```python
from build123d import *

# Parameters (mm, degrees)
SKETCH_R        = 4.075
PAD_DEPTH       = 10
SKETCH001_R     = 1.6
POCKET_DEPTH    = 10.501
POCKET001_DEPTH = 3
FILLET_R        = 3
FILLET001_R     = 1.5


with BuildPart() as part:
    # Sketch → Pad (new body)
    with BuildSketch(Plane.XY):
        with BuildLine():
            Line((20, -4.075), (20, -14.575))
            Line((20, -14.575), (-20, -14.575))
            Line((-20, -14.575), (-20, -4.075))
            Line((-20, -4.075), (-11.149975, -4.075))
            ThreePointArc((-11.149975, -4.075), (-8.268533, -2.881467), (-7.075, -2.5e-05))
            Line((-7.075, 0), (-7.075, -2.5e-05))
            ThreePointArc((7.075, 0), (0, 7.075), (-7.075, 0))
            Line((7.075, -2.5e-05), (7.075, 0))
            ThreePointArc((7.075, -2.5e-05), (8.268533, -2.881467), (11.149975, -4.075))
            Line((20, -4.075), (11.149975, -4.075))
        make_face()
        Circle(SKETCH_R, mode=Mode.SUBTRACT)
    extrude(amount=PAD_DEPTH)

    # Sketch001 (on Face6 of Pad) → Pocket (cut, through all)
    with BuildSketch(Plane(origin=(0, -4.075, 0), x_dir=(-1, 0, 0), z_dir=(0, 1, 0))):
        with Locations((-15.574988, 5)):
            Circle(SKETCH001_R)
        with Locations((15.574988, 5)):
            Circle(SKETCH001_R)
    extrude(amount=-POCKET_DEPTH, mode=Mode.SUBTRACT)

    # Sketch002 (on Face11 of Pocket) → Pocket001 (cut)
    with BuildSketch(Plane(origin=(0, -4.075, 0), x_dir=(-1, 0, 0), z_dir=(0, 1, 0))):
        Polygon((-15.574988, 8.233162), (-18.374988, 6.616581), (-18.374988, 3.383419), (-15.574988, 1.766838), (-12.774988, 3.383419), (-12.774988, 6.616581), align=None)
        Polygon((15.574988, 8.233162), (12.774988, 6.616581), (12.774988, 3.383419), (15.574988, 1.766838), (18.374988, 3.383419), (18.374988, 6.616581), align=None)
    extrude(amount=-POCKET001_DEPTH, mode=Mode.SUBTRACT)

    # Fillet
    fillet_edges = [part.edges().sort_by_distance(p)[0] for p in [
        (-20, -9.325, 0),
        (-20, -9.325, 10),
        (20, -9.325, 0),
        (20, -9.325, 10),
    ]]
    fillet(fillet_edges, radius=FILLET_R)

    # Fillet001
    fillet001_edges = [part.edges().sort_by_distance(p)[0] for p in [
        (-4.075, 0, 10),
        (-4.075, 0, 0),
    ]]
    fillet(fillet001_edges, radius=FILLET001_R)


solid = part.part
```
Read the model definition and answer for the solid it produces. Units are mm, in the model's axes. A direction names the side the tool comes from. Give positions to 0.01 mm unless a question says otherwise; leave off trailing zeros. Write each loop counter-clockwise with the first axis right and the second up, starting at its lowest first coordinate (ties: lowest second). Pieces come first, ordered by that corner, then holes. Notation, with made-up numbers: M 87.25,66.5 L 92.25,66.5 A9 ccw 92.25,76.5 Z; hole C 28.25,71 d7. An arc over 180 degrees is marked long. Put each result on its own line as item: value. Start each with the question number.
1. Each of these flat-tipped pins is pushed along its axis until it touches: pin 1 Ø1 at (y, z) = (-10, 9) entering from -X; pin 2 Ø4.5 at (x, z) = (-15, 4) entering from +Y (3 decimals); pin 3 Ø4.5 at (x, z) = (16, 5) entering from +Y (3 decimals). Where does it stop, or does it pass through?
2. For a pull along Z with two mould halves and no side action, classify faces 6 (the flat face through (0, -8, 10)), 7 (the flat face through (-20, -9, 5)), 8 (the flat face through (-14.155, -5.554, 2.586)) as released by +Z, released by -Z, zero draft, split by the parting line, or undercut.
3. The part is cut by section C-C, the plane x = 0. Give the vertices of the cut face in (y, z) (3 decimals), and give its area (3 significant figures).
4. The part is cut by section A-A, the plane z = 5. Give the number of separate pieces and of enclosed holes in the cut face, and give its area (3 significant figures).
5. The part is cut by section B-B, the plane y = -7.5. Give the vertices of the cut face in (x, z).
6. Consider line 1 along X through (y, z) = (-5, 4.5); line 2 along Y through (x, z) = (0, 4) (3 decimals); line 3 along Y through (x, z) = (-13.5, 3) (3 decimals). Determine where each line is inside the solid, lowest interval first.
7. Which of the six approach directions +Z, -Z, +X, -X, +Y, -Y give full straight-line access (tool end or side, diameter ignored) to faces 1 (the flat face through (16.995, -5.554, 2.586)), 2 (the flat face through (-17.6, -4.075, 2.7)), 3 (the cylindrical face through (19.14, -9.4, 9.1)), 4 (the flat face through (17.6, -4.075, 2.7)), 5 (the cylindrical face through (-17.053, -10.772, 4.387))?
Final values:
1. pin 1: stops at x = -19.6
1. pin 2: stops at y = -4.075
1. pin 3: stops at y = -7.075
2. face 6: released by +Z
2. face 7: zero draft
2. face 8: undercut
3. outline: M -14.575,0 L -5.575,0 A1.5 ccw -4.075,1.5 L -4.075,8.5 A1.5 ccw -5.575,10 L -14.575,10 Z; M 4.075,1.5 A1.5 ccw 5.575,0 L 7.075,0 L 7.075,10 L 5.575,10 A1.5 ccw 4.075,8.5 Z
3. area: 133 mm²
4. separate pieces: 3
4. enclosed holes: 1
4. area: 430 mm²
5. outline: M -20,3 A3 ccw -17,0 L 17,0 A3 ccw 20,3 L 20,7 A3 ccw 17,10 L -17,10 A3 ccw -20,7 Z; hole C -15.57,5 d3.2; hole C 15.57,5 d3.2
6. line 1: x = -20 to -18.37, -12.77 to 12.77, 18.37 to 20
6. line 2: y = -14.575 to -4.075, 4.075 to 7.075
6. line 3: y = -14.575 to -7.075
7. face 1: +Y
7. face 2: +Z, -Z, -X, +Y
7. face 3: +Z, +X, +Y, -Y
7. face 4: +Z, -Z, +X, +Y
7. face 5: +Y, -Y
